Could you check a few things on this model? Use its own coordinates, in mm. Face numbers are marked on the shaded views. A direction names the side the tool comes from. Give positions to 0.01 mm unless a question says otherwise; leave off trailing zeros. Write each loop counter-clockwise with the first axis right and the second up, starting at its lowest first coordinate (ties: lowest second). Pieces come first, ordered by that corner, then holes. Notation, with made-up numbers: (32.5, 15) - (90.5, 15) arc R18 ccw to (90.5, 33) - close; hole circle Ø1 at (-23, 64.5). An arc over 180 degrees is marked (long way). Answer as CSV lines item,"result". Start each with the question number.
Q1. On a 3-axis mill with a long thin cutter (end or side, diameter ignored), from which of +Z, -Z, +X, -X, +Y, -Y can I reach the whole of each face in a straight line? I mean the marked faces 4, 5, 6 and 7. Say none if no direction works.
Q2. Imagine slicing it at D-D on x = 10.25. List the corners of the cut face in (y, z) for me.
Q3. Will these pins go through, and if not, where does the flat tip stop? pin 1 Ø3 at (y, z) = (7.5, -1) entering from +X; pin 2 Ø6 at (x, z) = (12.5, 5.5) entering from -Y; pin 3 Ø4 at (x, y) = (10, -6.5) entering from +Z; pin 4 Ø1.5 at (x, y) = (14, -4.5) entering from -Z.
Q4. Imagine slicing it at B-B on y = -9. List the corners of the cut face in (x, z) for me, and give its area (3 significant figures).
Q5. We'd pull the mould along Y, two halves only. Please class the marked faces 1, 2 and 3: pulls with the +Y half, pulls with the -Y half, needs draft (parallel to the pull), parting line crosses it, or undercut.
Q6. Imagine slicing it at A-A on y = 0. List the corners of the cut face in (x, z) for me.
Q7. If I drill on line 1 along Y through (x, z) = (17, 0); line 2 along Y through (x, z) = (5, -6); line 3 along X through (y, z) = (7.25, 0.5), over which ranges is the centre line in solid material (lowest first)?
```python
from build123d import *

# Parameters (mm, degrees)
BASPROSKE_W         = 5.08
BASPROSKE_H         = 11.43
TOOTHCUT_DEPTH      = 17.943913361
TEETHCUTS_COUNT     = 16
TEETHCUTS_ANGLE     = 337.5
BORSKE_R            = 0.99949
BORE_DEPTH          = 50.8000508
SKETCH1_R           = 0.99949
BOSS_EXTRUDE1_DEPTH = 5.08
SKETCH2_R           = 4.269999969
BOSS_EXTRUDE2_DEPTH = 13.97
SKETCH3_R           = 2.65
CUT_EXTRUDE1_DEPTH  = 3.81


with BuildPart() as part:
    # BasProSke → Base-Revolve (revolve)
    with BuildSketch(Plane(origin=(0, 0, 0), x_dir=(1, 0, 0), z_dir=(0, 1, 0)), mode=Mode.PRIVATE) as base_revolve_sk:
        with Locations((2.54, 5.715)):
            Rectangle(BASPROSKE_W, BASPROSKE_H)
    revolve(base_revolve_sk.sketch.rotate(Axis((-10, 0, 0), (1, 0, 0)), 180), axis=Axis((-10, 0, 0), (1, 0, 0)))

    # TooCutSke → ToothCut (cut, through all)
    with BuildSketch(Plane(origin=(0, 0, 0), x_dir=(0, 0, -1), z_dir=(1, 0, 0))):
        with BuildLine():
            ThreePointArc((0.669851294, 8.559027882), (0, 8.5852), (-0.669851294, 8.559027882))
            ThreePointArc((-0.669851294, 8.559027882), (-1.058014649, 10.047160022), (-1.971359535, 11.284499579))
            ThreePointArc((-1.971359535, 11.284499579), (0, 11.4554), (1.971359535, 11.284499579))
            ThreePointArc((1.971359535, 11.284499579), (1.058014649, 10.047160022), (0.669851294, 8.559027882))
        make_face()
    toothcut = extrude(amount=TOOTHCUT_DEPTH, mode=Mode.SUBTRACT)

    # TeethCuts: ToothCut ×16 about axis
    teethcuts_axis = Axis((-10, 0, 0), (1, 0, 0))
    for i in range(1, TEETHCUTS_COUNT):
        add(toothcut.rotate(teethcuts_axis, i * TEETHCUTS_ANGLE / (TEETHCUTS_COUNT - 1)), mode=Mode.SUBTRACT)

    # BorSke → Bore (cut, symmetric)
    with BuildSketch(Plane(origin=(0, 0, 0), x_dir=(0, 0, -1), z_dir=(1, 0, 0))):
        with Locations(Location((0, 0, 0), (0, 0, 180))):
            Circle(BORSKE_R)
    extrude(amount=BORE_DEPTH, both=True, mode=Mode.SUBTRACT)

    # Sketch1 → Boss-Extrude1 (add)
    with BuildSketch(Plane(origin=(5.08, 0, 0), x_dir=(0, 0, -1), z_dir=(1, 0, 0))):
        Circle(SKETCH1_R)
    extrude(amount=-BOSS_EXTRUDE1_DEPTH)

    # Sketch2 → Boss-Extrude2 (add)
    with BuildSketch(Plane(origin=(5.08, 0, 0), x_dir=(0, 0, -1), z_dir=(1, 0, 0))):
        with Locations(Location((0, 0, 0), (0, 0, 180))):
            Circle(SKETCH2_R)
    extrude(amount=BOSS_EXTRUDE2_DEPTH)

    # Sketch3 → Cut-Extrude1 (cut)
    with BuildSketch(Plane(origin=(19.05, 0, 0), x_dir=(0, 0, -1), z_dir=(1, 0, 0))):
        Circle(SKETCH3_R)
    extrude(amount=-CUT_EXTRUDE1_DEPTH, mode=Mode.SUBTRACT)


solid = part.part
```
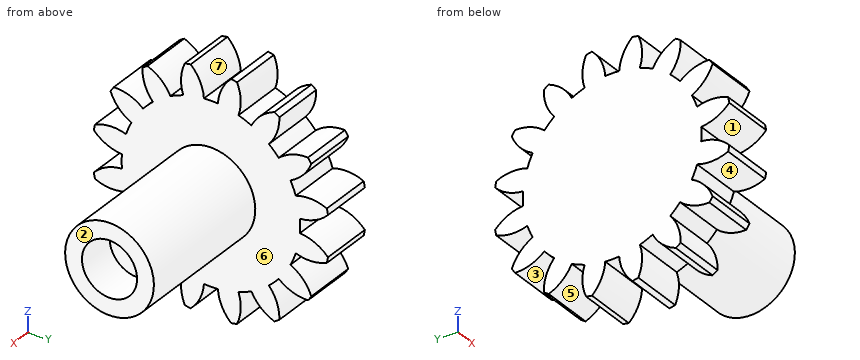
Conclusion:
1,face 4,"+X, -X"
1,face 5,"-Z, +X, -X"
1,face 6,"+X"
1,face 7,"+Z, +X, -X"
2,outline,"circle Ø8.54 at (0, 0)"
3,pin 1,"x = 5.08"
3,pin 2,"y = -3.46"
3,pin 3,"through"
3,pin 4,"z = -2.04"
4,outline,"(0, -6.58) - (5.08, -6.58) - (5.08, -4.97) - (0, -4.97) - close; (0, -2.85) - (5.08, -2.85) - (5.08, -0.72) - (0, -0.72) - close; (0, 0.72) - (5.08, 0.72) - (5.08, 2.85) - (0, 2.85) - close; (0, 4.97) - (5.08, 4.97) - (5.08, 6.58) - (0, 6.58) - close"
4,area,"38.0 mm^2"
5,face 1,"pulls with the -Y half"
5,face 2,"needs draft"
5,face 3,"undercut"
6,outline,"(0, -8.59) - (5.08, -8.59) - (5.08, -4.27) - (19.05, -4.27) - (19.05, -2.65) - (15.24, -2.65) - (15.24, 2.65) - (19.05, 2.65) - (19.05, 4.27) - (5.08, 4.27) - (5.08, 8.59) - (0, 8.59) - close"
7,line 1,"-4.27 to -2.65, 2.65 to 4.27"
7,line 2,"-9.62 to -7.1, -6.14 to 6.14, 7.1 to 9.62"
7,line 3,"0 to 5.08"
